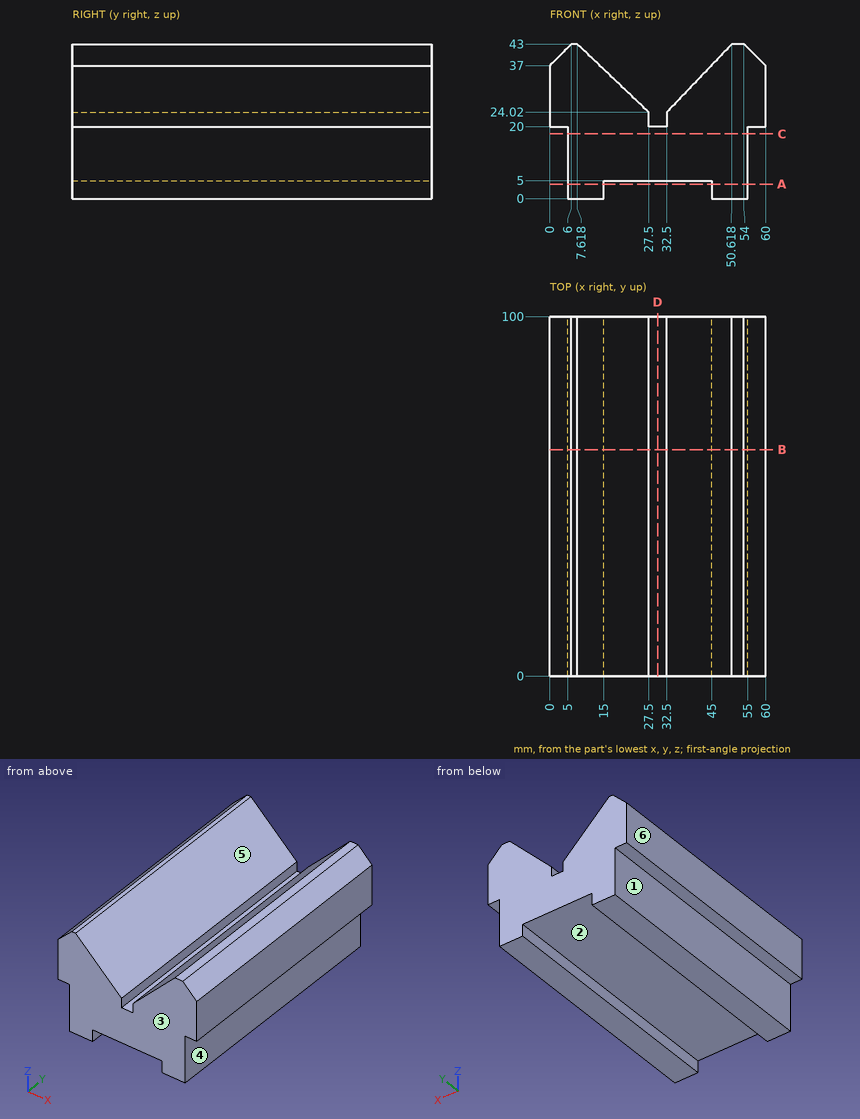
Here's the drawing with two shaded views (mm, measured from the low corner). I have some questions. A direction names the side the tool comes from. Give positions to 0.01 mm unless a question says otherwise; leave off trailing zeros. Order: outer loops, then holes, each group sorted by start corner. A loop starts at its lowest first (then second) coordinate and runs counter-clockwise, first axis right, second up. Notation, with made-up numbers: (39.5, -20) - (49.5, -20) arc R12 ccw to (49.5, 3) - close; hole circle Ø7 at (-5, 11). An arc over 180 degrees is marked (long way). Use a Markdown table: item, result. Add a question column.
Q1. If we section it at A-A on z = 4: Write out the boundary of the cut face in (x, y), plus the area to 3 significant figures.
Q2. If we section it at C-C on z = 18: Write out the boundary of the cut face in (x, y).
Q3. Please list where these lines run through material, in increasing order: line 1 along X through (y, z) = (73, 3); line 2 along X through (y, z) = (36, 22); line 3 along Z through (x, y) = (31, 86).
Q4. I'm going to push flat-ended pins straight in: pin 1 (9 mm diameter, centred on x = 33.5, y = 59, fed in from -Z); pin 2 (4 mm diameter, centred on y = 62.5, z = 3.5, fed in from -X); pin 3 (4 mm diameter, centred on x = 31, y = 38.5, fed in from +Z) (1 decimal). Where does each tip first touch, or does it pass through?
Q5. If we mould it in two halves opening along X, with no side actions, what happens to the marked faces 1, 2 and 3? For each: released by +X, released by -X, zero draft, split by the parting line, or undercut.
Q6. If we section it at B-B on y = 63: Write out the boundary of the cut face in (x, z), plus the area to 3 significant figures.
Q7. On a 3-axis mill with a long thin cutter (end or side, diameter ignored), from which of +Z, -Z, +X, -X, +Y, -Y can I reach the whole of each face in a straight line? I mean the marked faces 4, 5 and 6. Say none if no direction works.
Q8. If we section it at D-D on x = 30: Write out the boundary of the cut face in (y, z).
Answers follow:
| question | item | result |
|---|---|---|
| 1 | outline | (5, 0) - (15, 0) - (15, 100) - (5, 100) - close; (45, 0) - (55, 0) - (55, 100) - (45, 100) - close |
| 1 | area | 2,000 mm^2 |
| 2 | outline | (5, 0) - (55, 0) - (55, 100) - (5, 100) - close |
| 3 | line 1 | x = 5 to 15, 45 to 55 |
| 3 | line 2 | x = 0 to 27.5, 32.5 to 60 |
| 3 | line 3 | z = 5 to 20 |
| 4 | pin 1 | stops at z = 5 |
| 4 | pin 2 | stops at x = 5 |
| 4 | pin 3 | stops at z = 24.5 |
| 5 | face 1 | released by -X |
| 5 | face 2 | undercut |
| 5 | face 3 | zero draft |
| 6 | outline | (0, 20) - (5, 20) - (5, 0) - (15, 0) - (15, 5) - (45, 5) - (45, 0) - (55, 0) - (55, 20) - (60, 20) - (60, 37) - (54, 43) - (50.62, 43) - (32.5, 24.02) - (32.5, 20) - (27.5, 20) - (27.5, 24.02) - (7.62, 43) - (6, 43) - (0, 37) - close |
| 6 | area | 1,720 mm^2 |
| 7 | face 4 | -Z, +X, +Y, -Y |
| 7 | face 5 | +Z, +Y, -Y |
| 7 | face 6 | +Z, -Z, -X, +Y, -Y |
| 8 | outline | (0, 5) - (100, 5) - (100, 20) - (0, 20) - close |
